Can you work these out from the model? Positions are in its coordinate system, mm. A direction names the side the tool comes from. Give positions to 0.01 mm unless a question says otherwise; leave off trailing zeros. Loops run counter-clockwise (first coordinate to the right, second up) from the corner with the lowest first, then second, coordinate; pieces in that order, holes last. Notation, with made-up numbers: M 43.25,-39.5 L 48.25,-39.5 A20 cw 48.25,-13.5 Z; hole C 27,-4.5 d8. An arc over 180 degrees is marked long. Put each result on its own line as item: value. Start each with the question number.
1) Imagine slicing it at A-A (z = -48). Write out the boundary of the cut face in (x, y), then the cut area to 3 significant figures.
2) Imagine slicing it at D-D (x = -6.5). Write out the boundary of the cut face in (y, z), then the cut area to 3 significant figures.
3) Imagine slicing it at C-C (y = 0.15). Write out the boundary of the cut face in (x, z).
4) Imagine slicing it at B-B (x = -9). Write out the boundary of the cut face in (y, z).
5) Please list where these lines run through material, in increasing order: line 1 along Z through (x, y) = (-6.75, 0.6); line 2 along Z through (x, y) = (-7, 0.85); line 3 along X through (y, z) = (0.4, -42.75). Write a range as from..to.
6) For faces 1 (the flat face through (-3.038, 0.5, -35)), 2 (the cylindrical face through (-7.845, 0.493, -34.46)), which set-ups out of +Z, -Z, +X, -X, +Y, -Y let a thin tool reach every point of the face, with its end or its side?
7) If we mould it in two halves opening along X, with no side actions, what happens to faces 3 (the cylindrical face through (-1.949, 0.493, -33.522)), 4 (the cylindrical face through (-4.14, 0.49, -49.89)), 5 (the cylindrical face through (-4.15, 0.493, -48.966))? For each: +X half, -X half, draft (parallel to the pull), parting line (faces both ways), or undercut.
Autodesk Inventor part; units mm, degrees
ref_plane "YZ Plane" through (0, 0, 0) normal (1, 0, 0) x (0, 1, 0)
ref_plane "XZ Plane" through (0, 0, 0) normal (0, 1, 0) x (-1, 0, 0)
ref_plane "XY Plane" through (0, 0, 0) normal (0, 0, 1) x (1, 0, 0)
sketch "Sketch1" plane through (0, 0, 0) normal (0, 1, 0) x (-1, 0, 0)
  line L0 (4.788, -33.3618) -> (4.788, -36.6836)
  line L1 (8.1671, -36.2479) -> (8.1671, -35.4556)
  line L2 (-0.2231, -35.4067) -> (-0.2231, -36.199)
  line L3 (3.0381, -36.6804) -> (3.0381, -33.3586)
  circle A0 centre (6.4671, -35.4556) radius 0.85
  circle A1 centre (1.4769, -35.4067) radius 0.85
  arc A2 (3.0381, -36.6804) -> (4.788, -36.6836) centre (3.9019, -42.7951) ccw
  arc A3 (7.028, -33.8508) -> (4.788, -33.3618) centre (3.9019, -42.7951) ccw
  arc A4 (8.1671, -35.4556) -> (7.028, -33.8508) centre (6.4671, -35.4556) ccw
  arc A5 (8.1671, -36.2479) -> (8.6017, -37.4732) centre (9.8649, -36.3356) ccw
  arc A6 (-0.7978, -37.4732) -> (8.6017, -37.4732) centre (3.9019, -42.7951) ccw
  arc A7 (-0.7978, -37.4732) -> (-0.2231, -36.199) centre (-1.9231, -36.199) ccw
  arc A8 (0.9161, -33.8019) -> (-0.2231, -35.4067) centre (1.4769, -35.4067) ccw
  arc A9 (3.0381, -33.3586) -> (0.9161, -33.8019) centre (3.9019, -42.7951) ccw
  point P0 (0, 0)
  dimension "d0" = 0
  dimension "d1" = 0
  dimension "d2" = 0
  dimension "d3" = 0
  dimension "d4" = 6.1754
  dimension "d5" = 7.1
  dimension "d6" = 1.7
  dimension "d7" = 1.7
  dimension "d8" = 1.7
  dimension "d9" = 1.7
  dimension "d10" = 1.7
  dimension "d11" = 1.7
  dimension "d12" = 9.476
  dimension "d13" = 9.4748
  dimension "d14" = 1.7499
extrude "Extrusion1" add sketch "Sketch1" along normal blind 1
properties part number "49-01-004"
Recorded:
1. outline: M -8.73,0 L -7.23,0 L -7.23,1 L -8.73,1 Z; M -0.58,0 L 0.93,0 L 0.93,1 L -0.58,1 Z
1. area: 3.01 mm²
2. outline: M 0,-49.4 L 1,-49.4 L 1,-48.4 L 0,-48.4 Z; M 0,-37.19 L 1,-37.19 L 1,-36.3 L 0,-36.3 Z; M 0,-34.61 L 1,-34.61 L 1,-33.68 L 0,-33.68 Z
2. area: 2.82 mm²
3. outline: M -8.6,-37.47 A7.1 ccw long 0.8,-37.47 A1.7 cw 0.22,-36.2 L 0.22,-35.41 A1.7 ccw -0.92,-33.8 A9.47 ccw -3.04,-33.36 L -3.04,-36.68 A6.18 cw long -4.79,-36.68 L -4.79,-33.36 A9.47 ccw -7.03,-33.85 A1.7 ccw -8.17,-35.46 L -8.17,-36.25 A1.7 cw Z; hole C -6.47,-35.46 d1.7; hole C -1.48,-35.41 d1.7
4. outline: M 0,-47.74 L 1,-47.74 L 1,-46.28 L 0,-46.28 Z; M 0,-39.31 L 1,-39.31 L 1,-37.85 L 0,-37.85 Z
5. line 1: -49.3..-48.27, -37.32..-36.26, -34.65..-33.76
5. line 2: -49.18..-48.14, -37.45..-36.12, -34.79..-33.84
5. line 3: -11..-10.08, 2.27..3.2
6. face 1: +Z, +Y, -Y
6. face 2: +Z, -X, +Y, -Y
7. face 3: +X half
7. face 4: parting line
7. face 5: undercut
